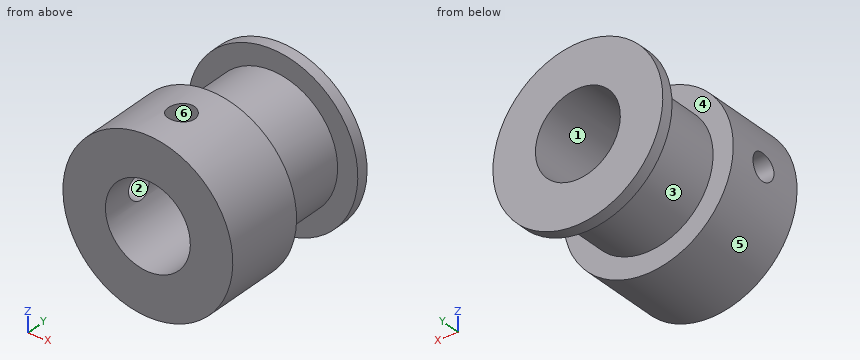
from build123d import *

# Parameters (mm, degrees)
M3_GEWINDEBOHRUNG1_REACH  = 26
M3_GEWINDEBOHRUNG1_BORE_R = 1.25
KREISMUSTER1_COUNT        = 2
KREISMUSTER1_ANGLE        = 90


with BuildPart() as part:
    # Skizze1 → Rotation1 (revolve)
    with BuildSketch(Plane.XY, mode=Mode.PRIVATE) as rotation1_sk:
        Polygon((-4, 16), (-4, 0), (-8, 0), (-8, 7.6), (-6.1, 7.6), (-6.1, 14.9), (-8, 14.9), (-8, 16), align=None)
    revolve(rotation1_sk.sketch.rotate(Axis((0, 0, 0), (0, 1, 0)), 270), axis=Axis((0, 0, 0), (0, 1, 0)))

    # M3 Gewindebohrung1 bore → M3 Gewindebohrung1 (cut, up to next)
    with BuildSketch(Plane.XY.offset(8), mode=Mode.PRIVATE) as m3_gewindebohrung1_sk1:
        with Locations((0, 4)):
            Circle(M3_GEWINDEBOHRUNG1_BORE_R)
    m3_gewindebohrung1_tool1 = extrude(m3_gewindebohrung1_sk1.sketch, amount=-M3_GEWINDEBOHRUNG1_REACH, mode=Mode.PRIVATE) & part.part
    m3_gewindebohrung1 = m3_gewindebohrung1_tool1.solids().sort_by_distance((0, 4, 8))[0]
    add(m3_gewindebohrung1, mode=Mode.SUBTRACT)

    # Kreismuster1: M3 Gewindebohrung1 ×2 about axis
    kreismuster1_axis = Axis((0, 0, 0), (0, -1, 0))
    for i in range(1, KREISMUSTER1_COUNT):
        add(m3_gewindebohrung1.rotate(kreismuster1_axis, i * KREISMUSTER1_ANGLE / (KREISMUSTER1_COUNT - 1)), mode=Mode.SUBTRACT)


solid = part.part
The model under review builds one solid part; all positions refer to its coordinate system, in mm. Face numbers are marked on the shaded views. A direction names the side the tool comes from. Coordinates: 2 decimals unless noted, no trailing zeros. Write each loop counter-clockwise with the first axis right and the second up, starting at its lowest first coordinate (ties: lowest second). Pieces come first, ordered by that corner, then holes. Notation, with made-up numbers: (27.5, 87) - (31.5, 87) arc R29 ccw to (31.5, 118) - close; hole circle Ø1 at (43.25, -32). An arc over 180 degrees is marked (long way). Answer as a JSON object with one key per item and string values. Group by question number.
1. Add section D-D (y = 4). Give the boundary of the cut face in (x, z).
2. Add section C-C (z = -6.5). Give the boundary of the cut face in (x, y).
3. Add section B-B (z = 0). Give the boundary of the cut face in (x, y).
4. Clearance check with flat-ended pins moving along their axes: pin 1 Ø2 at (y, z) = (4, 0) entering from -X; pin 2 Ø5 at (x, y) = (-6, 6.5) entering from -Z; pin 3 Ø5 at (x, z) = (0, 0) entering from -Y. State where each tip first meets the part, or that it passes through.
5. Machinability: for the marked faces 4, 5 and 6, which of the approach directions +Z, -Z, +X, -X, +Y, -Y give a long, thin tool a straight path to every point of the face, cutting with its end or side? Answer none if there is none.
6. Mouldability with a two-part tool opening along X and no side actions: class the marked faces 1, 2 and 3 as pulls with the +X half, pulls with the -X half, needs draft (parallel to the pull), parting line crosses it, or undercut.
7. To check wall thickness, follow probe 1 along Y at (x, z) = (0, 6.25); probe 2 along Y at (x, z) = (0, 5.8); probe 3 along Y at (x, z) = (5, -4.5). State the ranges of each line that lie inside material, in increasing order.
8. Add section A-A (x = 0). Give the boundary of the cut face in (y, z), plus the area to 3 significant figures.
Findings:
{
 "1": {"outline": "(-7.9, -1.25) arc R8 ccw (long way) to (1.25, 7.9) - (1.25, 3.8) arc R4 cw (long way) to (-3.8, -1.25) - close; (-7.9, 1.25) - (-3.8, 1.25) arc R4 cw to (-1.25, 3.8) - (-1.25, 7.9) arc R8 ccw to start"},
 "2": {"outline": "(-4.66, 0) - (4.66, 0) - (4.66, 7.6) - (-4.66, 7.6) - close; (-4.66, 14.9) - (4.66, 14.9) - (4.66, 16) - (-4.66, 16) - close"},
 "3": {"outline": "(-8, 0) - (-4, 0) - (-4, 2.75) - (-8, 2.75) - close; (-8, 5.25) - (-4, 5.25) - (-4, 16) - (-8, 16) - (-8, 14.9) - (-6.1, 14.9) - (-6.1, 7.6) - (-8, 7.6) - close; (4, 0) - (8, 0) - (8, 7.6) - (6.1, 7.6) - (6.1, 14.9) - (8, 14.9) - (8, 16) - (4, 16) - close"},
 "4": {"pin 1": "x = 3.87", "pin 2": "z = -7.19", "pin 3": "through"},
 "5": {"face 4": "none", "face 5": "+Y, -Y", "face 6": "+Z"},
 "6": {"face 1": "undercut", "face 2": "needs draft", "face 3": "parting line crosses it"},
 "7": {"probe 1": "0 to 2.75, 5.25 to 7.6, 14.9 to 16", "probe 2": "0 to 2.75, 5.25 to 16", "probe 3": "0 to 7.6, 14.9 to 16"},
 "8": {"outline": "(0, -8) - (7.6, -8) - (7.6, -6.1) - (14.9, -6.1) - (14.9, -8) - (16, -8) - (16, -4) - (0, -4) - close; (0, 4) - (2.75, 4) - (2.75, 8) - (0, 8) - close; (5.25, 4) - (16, 4) - (16, 8) - (14.9, 8) - (14.9, 6.1) - (7.6, 6.1) - (7.6, 8) - (5.25, 8) - close", "area": "90.3 mm²"}
}
